Part model, mm, in its own coordinate system. A direction names the side the tool comes from. Round coordinates to 2 decimals unless told otherwise and drop trailing zeros. Order: outer loops, then holes, each group sorted by start corner. A loop starts at its lowest first (then second) coordinate and runs counter-clockwise, first axis right, second up. Notation, with made-up numbers: M -9,22 L 34,22 A23 ccw 34,51 Z; hole C -16.5,33.25 d1. An arc over 180 degrees is marked long. Write each question's results on one line, items separated by ' | '. Start each with the question number.
1. Which spindle directions (+Z, -Z, +X, -X, +Y, -Y) get a long thin tool onto all of the face, cutting with end or side? Do faces 1 (the face through (1.532, -3.695, 18.662)), 2 (the face through (0.471, 5.426, 18.864)), 3 (the face through (0, -3, 0)). Say none if no direction does.
2. Probe L1, parallel to Y at x = 0, z = 9.25; L2, parallel to Y at x = -3, z = 13; L3, parallel to Z at x = -2, y = -2.5. List the from-to ranges inside material, lowest first. Write a range as [from, to].
3. Drop flat-ended pins along their axis: pin 1 Ø5 at (x, z) = (-3.5, 9) entering from +Y; pin 2 Ø2.5 at (x, y) = (1, -1) entering from +Z; pin 3 Ø1.5 at (x, z) = (4, 8.5) entering from -Y. Give the stop position or say it passes through.
4. Band-saw the part on A-A, the plane y = 0. List the corners of the cut face in (x, z), then the cut area to 4 significant figures.
5. Band-saw the part on B-B, the plane x = 0. List the corners of the cut face in (y, z).
6. Two-plate mould, pull along Y, no slides. Class faces 4 (the face through (0.471, 4.622, 3.864)), 5 (the face through (6.466, 2.681, 12.325)), 6 (the face through (-0.751, -2.385, 6.162)): +Y half, -Y half, draft (parallel to the pull), parting line (faces both ways), or undercut.
7. Band-saw the part on C-C, the plane z = 2.5. List the corners of the cut face in (x, y).
8. Band-saw the part on D-D, the plane x = -2. List the corners of the cut face in (y, z).
Autodesk Inventor part; units mm, degrees
ref_plane "YZ Plane" through (0, 0, 0) normal (1, 0, 0) x (0, 1, 0)
ref_plane "XZ Plane" through (0, 0, 0) normal (0, 1, 0) x (-1, 0, 0)
ref_plane "XY Plane" through (0, 0, 0) normal (0, 0, 1) x (1, 0, 0)
sketch "Sketch1" plane through (0, 0, 0) normal (0, 0, 1) x (1, 0, 0)
  circle A0 centre (0, 0) radius 7
  dimension "d0" = 14
extrude "Extrusion1" add sketch "Sketch1" along normal blind 25
sketch "Sketch3" plane through (0, 0, 25) normal (0, 0, 1) x (1, 0, 0)
  circle A0 centre (0, 0) radius 7
hole "Hole1" at (0, 0, 25) direction (0, 0, -1) diameter 5 end through all counterbore diameter 8 counterbore depth 12.5
sketch "Sketch4" plane through (0, 0, 0) normal (0, 1, 0) x (-1, 0, 0)
  line L0 (7, 25) -> (-7, 25)
  line L1 (7, 0) -> (-7, 0)
  point P0 (0, 0)
  point P1 (0, 20)
  point P2 (0, 5)
  dimension "d10" = 5
  dimension "d11" = 5
hole "Hole2" at (0, 0, 20) at (0, 0, 5) direction (0, 1, 0) diameter 2.459 depth 8.8 tip angle 118
properties part number "10-03-05 Hub"
Solution:
1) face 1: +Z | face 2: +Y | face 3: -Z, +X, -X, +Y, -Y
2) L1: [-7, -2.5], [2.5, 7] | L2: [-6.32, -2.65], [2.65, 6.32] | L3: [0, 12.5]
3) pin 1: y = 6.93 | pin 2: z = 12.5 | pin 3: y = -6.2
4) outline: M -7,0 L -2.5,0 L -2.5,12.5 L -4,12.5 L -4,25 L -7,25 Z; M 2.5,0 L 7,0 L 7,25 L 4,25 L 4,12.5 L 2.5,12.5 Z | area: 187.5 mm^2
5) outline: M -7,0 L -2.5,0 L -2.5,12.5 L -4,12.5 L -4,25 L -7,25 Z; M 2.5,0 L 7,0 L 7,3.77 L 2.5,3.77 Z; M 2.5,6.23 L 7,6.23 L 7,18.77 L 4,18.77 L 4,12.5 L 2.5,12.5 Z; M 4,21.23 L 7,21.23 L 7,25 L 4,25 Z
6) face 4: draft | face 5: parting line | face 6: undercut
7) outline: C 0,0 d14; hole C 0,0 d5
8) outline: M -6.71,0 L -1.5,0 L -1.5,12.5 L -3.46,12.5 L -3.46,25 L -6.71,25 Z; M 1.5,0 L 6.71,0 L 6.71,25 L 3.46,25 L 3.46,12.5 L 1.5,12.5 Z
